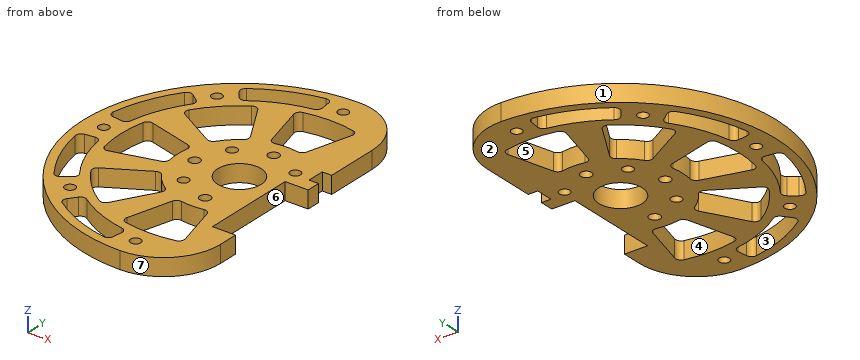
```python
from build123d import *

# Parameters (mm, degrees)
SKETCH1_R                = 57.5
SKETCH1_R_2              = 1.89865
SKETCH1_R_3              = 1.9939
SKETCH1_R_4              = 8
BOSS_EXTRUDE1_DEPTH      = 6.35
CUT_EXTRUDE1_DEPTH       = 82.564836173
SKETCH3_W                = 6.35
SKETCH3_H                = 80
CUT_EXTRUDE3_DEPTH       = 82.564836173
CUT_EXTRUDE5_DEPTH       = 82.564836173
CUT_EXTRUDE7_DEPTH       = 82.564836173
FILLET1_R                = 2
CIRPATTERN1_COUNT        = 8
FILLET1_OF_CIRPATTERN1_R = 2
CUT_EXTRUDE8_DEPTH       = 82.564836173
FILLET2_R                = 2
CIRPATTERN2_COUNT        = 8
FILLET2_OF_CIRPATTERN2_R = 2


with BuildPart() as part:
    # Sketch1 → Boss-Extrude1 (new body)
    with BuildSketch(Plane.XY):
        Circle(SKETCH1_R)
        with Locations((45.315389352, 21.130913087)):
            Circle(SKETCH1_R_2, mode=Mode.SUBTRACT)
        with Locations((49.978847504, 1.454235937)):
            Circle(SKETCH1_R_3, mode=Mode.SUBTRACT)
        Circle(SKETCH1_R_4, mode=Mode.SUBTRACT)
        with Locations((46.467376211, -18.460307366)):
            Circle(SKETCH1_R_3, mode=Mode.SUBTRACT)
        with Locations((0, -16.5)):
            Circle(SKETCH1_R_3, mode=Mode.SUBTRACT)
        with Locations((0, -50)):
            Circle(SKETCH1_R_2, mode=Mode.SUBTRACT)
        with Locations((-16.5, 0)):
            Circle(SKETCH1_R_3, mode=Mode.SUBTRACT)
        with Locations((-11.66726189, -11.66726189)):
            Circle(SKETCH1_R_2, mode=Mode.SUBTRACT)
        with Locations((0, 16.5)):
            Circle(SKETCH1_R_3, mode=Mode.SUBTRACT)
        with Locations((-11.66726189, 11.66726189)):
            Circle(SKETCH1_R_2, mode=Mode.SUBTRACT)
        with Locations((11.66726189, 11.66726189)):
            Circle(SKETCH1_R_2, mode=Mode.SUBTRACT)
        with Locations((-35.355339059, -35.355339059)):
            Circle(SKETCH1_R_2, mode=Mode.SUBTRACT)
        with Locations((-50, 0)):
            Circle(SKETCH1_R_2, mode=Mode.SUBTRACT)
        with Locations((-35.355339059, 35.355339059)):
            Circle(SKETCH1_R_2, mode=Mode.SUBTRACT)
        with Locations((0, 50)):
            Circle(SKETCH1_R_2, mode=Mode.SUBTRACT)
        with Locations((35.355339059, -35.355339059)):
            Circle(SKETCH1_R_2, mode=Mode.SUBTRACT)
    extrude(amount=BOSS_EXTRUDE1_DEPTH)

    # Sketch2 → Cut-Extrude1 (cut, through all)
    with BuildSketch(Plane.XY):
        Polygon((12.5, -29.35), (41, -29.35), (41, 10.65), (44.5, 10.65), (44.5, 17), (41, 17), (41, 32), (21, 32), (21, 17), (17.5, 17), (17.5, 10.65), (21, 10.65), (21, 5.65), (12.5, 5.65), align=None)
    extrude(amount=CUT_EXTRUDE1_DEPTH, mode=Mode.SUBTRACT)

    # Sketch3 → Cut-Extrude3 (cut, through all)
    with BuildSketch(Plane(origin=(0, 0, 0), x_dir=(-1, 0, 0), z_dir=(0, 0, -1))):
        with Locations((-31, 32)):
            Rectangle(SKETCH3_W, SKETCH3_H)
    extrude(amount=-CUT_EXTRUDE3_DEPTH, mode=Mode.SUBTRACT)

    # Sketch4 → Cut-Extrude5 (cut, through all)
    with BuildSketch(Plane.XY):
        with BuildLine():
            Line((21, -36.500002949), (21, -5.372089924))
            Line((21, -5.372089924), (24.175, -5.411516926))
            Line((24.175, -5.411516926), (24.175, -57.5))
            Line((24.175, -57.5), (2.949e-06, -57.5))
            ThreePointArc((2.949e-06, -57.5), (14.849243269, -51.349243269), (21, -36.500002949))
        make_face()
        with BuildLine():
            Line((2.949e-06, 57.5), (24.175, 57.5))
            Line((24.175, 57.5), (24.175, 5.411516926))
            Line((24.175, 5.411516926), (21, 5.372089924))
            Line((21, 5.372089924), (21, 36.500002949))
            ThreePointArc((21, 36.500002949), (14.849243269, 51.349243269), (2.949e-06, 57.5))
        make_face()
    extrude(amount=CUT_EXTRUDE5_DEPTH, mode=Mode.SUBTRACT)


with BuildPart() as cut_extrude5_kept_piece:
    # of the separate pieces the step leaves, the one the design keeps (cut_extrude5_pieces_kept)
    add(part.part.solids().sort_by_distance((2.949e-06, 57.5, 0))[0])

    # Sketch6 → Cut-Extrude7 (cut, through all)
    with BuildSketch(Plane.XY.offset(6.35)):
        with BuildLine():
            Line((-42.162662318, -11.297451319), (-22.071405131, -5.914015181))
            ThreePointArc((-22.071405131, -5.914015181), (-22.85, 0), (-22.071405131, 5.914015181))
            Line((-22.071405131, 5.914015181), (-42.162662318, 11.297451319))
            ThreePointArc((-42.162662318, 11.297451319), (-43.65, 0), (-42.162662318, -11.297451319))
        make_face()
    cut_extrude7 = extrude(amount=-CUT_EXTRUDE7_DEPTH, mode=Mode.SUBTRACT)

    # Fillet1
    fillet1_edges = [cut_extrude5_kept_piece.edges().sort_by_distance(p)[0] for p in [
        (-22.071405131, 5.914015181, 3.175),
        (-22.071405131, -5.914015181, 3.175),
        (-42.162662318, -11.297451319, 3.175),
        (-42.162662318, 11.297451319, 3.175),
    ]]
    fillet(fillet1_edges, radius=FILLET1_R)

    # CirPattern1: Cut-Extrude7 ×8 about axis, 3 skipped
    cirpattern1_axis = Axis((0, 0, 0), (0, 0, -1))
    add([cut_extrude7.rotate(cirpattern1_axis, i * 360 / CIRPATTERN1_COUNT) for i in range(1, CIRPATTERN1_COUNT) if i not in (3, 4, 5)], mode=Mode.SUBTRACT)

    # Fillet1 of CirPattern1
    fillet1_of_cirpattern1_edges = [cut_extrude5_kept_piece.edges().sort_by_distance(p)[0] for p in [
        (-11.425, 19.788680476, 3.175),
        (-19.788680476, 11.425, 3.175),
        (-37.802008875, 21.825, 3.175),
        (-21.825, 37.802008875, 3.175),
        (5.914015181, 22.071405131, 3.175),
        (-5.914015181, 22.071405131, 3.175),
        (-11.297451319, 42.162662318, 3.175),
        (11.297451319, 42.162662318, 3.175),
        (-5.914015181, -22.071405131, 3.175),
        (5.914015181, -22.071405131, 3.175),
        (11.297451319, -42.162662318, 3.175),
        (-11.297451319, -42.162662318, 3.175),
        (-19.788680476, -11.425, 3.175),
        (-11.425, -19.788680476, 3.175),
        (-21.825, -37.802008875, 3.175),
        (-37.802008875, -21.825, 3.175),
    ]]
    fillet(fillet1_of_cirpattern1_edges, radius=FILLET1_OF_CIRPATTERN1_R)

    # Sketch7 → Cut-Extrude8 (cut, through all)
    with BuildSketch(Plane.XY.offset(6.35)):
        with BuildLine():
            Line((-43.098920211, 33.070964631), (-37.148770159, 28.505253913))
            ThreePointArc((-37.148770159, 28.505253913), (-43.26065911, 17.91915172), (-46.424405634, 6.111888951))
            Line((-46.424405634, 6.111888951), (-53.860242094, 7.090835392))
            ThreePointArc((-53.860242094, 7.090835392), (-50.189755604, 20.789277463), (-43.098920211, 33.070964631))
        make_face()
    cut_extrude8 = extrude(amount=-CUT_EXTRUDE8_DEPTH, mode=Mode.SUBTRACT)

    # Fillet2
    fillet2_edges = [cut_extrude5_kept_piece.edges().sort_by_distance(p)[0] for p in [
        (-53.860242094, 7.090835392, 3.175),
        (-43.098920211, 33.070964631, 3.175),
        (-37.148770159, 28.505253913, 3.175),
        (-46.424405634, 6.111888951, 3.175),
    ]]
    fillet(fillet2_edges, radius=FILLET2_R)

    # CirPattern2: Cut-Extrude8 ×8 about axis, 4 skipped
    cirpattern2_axis = Axis((0, 0, 0), (0, 0, -1))
    add([cut_extrude8.rotate(cirpattern2_axis, i * 360 / CIRPATTERN2_COUNT) for i in range(1, CIRPATTERN2_COUNT) if i not in (2, 3, 4, 5)], mode=Mode.SUBTRACT)

    # Fillet2 of CirPattern2
    fillet2_of_cirpattern2_edges = [cut_extrude5_kept_piece.edges().sort_by_distance(p)[0] for p in [
        (-33.070964631, 43.098920211, 3.175),
        (-7.090835392, 53.860242094, 3.175),
        (-6.111888951, 46.424405634, 3.175),
        (-28.505253913, 37.148770159, 3.175),
        (-7.090835392, -53.860242094, 3.175),
        (-33.070964631, -43.098920211, 3.175),
        (-28.505253913, -37.148770159, 3.175),
        (-6.111888951, -46.424405634, 3.175),
        (-43.098920211, -33.070964631, 3.175),
        (-53.860242094, -7.090835392, 3.175),
        (-46.424405634, -6.111888951, 3.175),
        (-37.148770159, -28.505253913, 3.175),
    ]]
    fillet(fillet2_of_cirpattern2_edges, radius=FILLET2_OF_CIRPATTERN2_R)


solid = cut_extrude5_kept_piece.part
```
Source: CAD feature listing. Evaluate the final solid. Frame: model axes, mm. Face numbers are marked on the shaded views. A direction names the side the tool comes from. Give positions to 0.01 mm unless a question says otherwise; leave off trailing zeros. Loops run counter-clockwise (first coordinate to the right, second up) from the corner with the lowest first, then second, coordinate; pieces in that order, holes last. Notation, with made-up numbers: (-10, 5) -> (43, 5) arc R16 cw to (43, 30) -> close; hole circle Ø3 at (-40, 78). An arc over 180 degrees is marked (long way). Put each result on its own line as item: value. Start each with the question number.
1) Cut plane C-C (y = -50). Return loops of the section in (x, z).
2) Contact query for flat-ended pins moving along their axis: P1, Ø5, axis at x = 0, y = 50, coming from the -Z side; P2, Ø1.9, axis at y = -6, z = 3, coming from the +X side; P3, Ø3, axis at x = -28, z = 1.5, coming from the +Y side; P4, Ø1, axis at x = 18.5, z = 2.5, coming from the +Y side. Output: stop coordinate, or through.
3) Material intervals for probe 1 along X at (y, z) = (-17, 0.5); probe 2 along Y at (x, z) = (-29, 0.5); probe 3 along X at (y, z) = (-19.5, 4.75) (3 decimals), sorted ascending.
4) Cut plane D-D (x = 16). Return loops of the section in (y, z).
5) Draft query along X for the marked faces 1, 2, 3 and 4. Return one class per face: released by +X, released by -X, zero draft, split by the parting line, or undercut.
6) Reachability of the marked faces 5, 6 and 7 from +Z, -Z, +X, -X, +Y, -Y: full face, straight path, thin tool, end or side. Return the list, or none.
7) Cut plane B-B (x = -25.5). Return loops of the section in (y, z), then the cut area to 3 significant figures.
8) Cut plane A-A (y = 0). Return loops of the section in (x, z), then the cut area to 3 significant figures.
Results are:
1. outline: (-28.39, 0) -> (-21.24, 0) -> (-21.24, 6.35) -> (-28.39, 6.35) -> close; (-6.58, 0) -> (-1.9, 0) -> (-1.9, 6.35) -> (-6.58, 6.35) -> close; (1.9, 0) -> (16.09, 0) -> (16.09, 6.35) -> (1.9, 6.35) -> close
2. P1: stops at z = 0
2. P2: stops at x = 12.5
2. P3: stops at y = 51.03
2. P4: stops at y = 47.32
3. probe 1: x = -54.93 to -51.6, -43.63 to -29.44, -15.27 to -1.93, 1.93 to 12.5
3. probe 2: y = -49.65 to -45.94, -38.13 to -32.62, -16.74 to -7.77, 7.77 to 16.74, 32.62 to 38.13, 45.94 to 49.65
3. probe 3: x = -54.093 to -50.705, -42.571 to -33.775, -12.357 to 12.5
4. outline: (-50.1, 0) -> (-29.35, 0) -> (-29.35, 6.35) -> (-50.1, 6.35) -> close; (5.65, 0) -> (50.1, 0) -> (50.1, 6.35) -> (5.65, 6.35) -> close
5. face 1: released by -X
5. face 2: zero draft
5. face 3: undercut
5. face 4: undercut
6. face 5: +Z, -Z
6. face 6: +Z, -Z, +X
6. face 7: +Z, -Z, +X, -Y
7. outline: (-51.54, 0) -> (-47.97, 0) -> (-47.97, 6.35) -> (-51.54, 6.35) -> close; (-39.27, 0) -> (-35.43, 0) -> (-35.43, 6.35) -> (-39.27, 6.35) -> close; (-14.72, 0) -> (-6.83, 0) -> (-6.83, 6.35) -> (-14.72, 6.35) -> close; (6.83, 0) -> (14.72, 0) -> (14.72, 6.35) -> (6.83, 6.35) -> close; (35.43, 0) -> (39.27, 0) -> (39.27, 6.35) -> (35.43, 6.35) -> close; (47.97, 0) -> (51.54, 0) -> (51.54, 6.35) -> (47.97, 6.35) -> close
7. area: 194 mm2
8. outline: (-57.5, 0) -> (-51.9, 0) -> (-51.9, 6.35) -> (-57.5, 6.35) -> close; (-48.1, 0) -> (-43.65, 0) -> (-43.65, 6.35) -> (-48.1, 6.35) -> close; (-22.85, 0) -> (-18.49, 0) -> (-18.49, 6.35) -> (-22.85, 6.35) -> close; (-14.51, 0) -> (-8, 0) -> (-8, 6.35) -> (-14.51, 6.35) -> close; (8, 0) -> (12.5, 0) -> (12.5, 6.35) -> (8, 6.35) -> close
8. area: 161 mm2
